```python
from build123d import *

# Parameters (mm, degrees)
ZAAWANSOWANYOTW_R1_START       = 2
ZAAWANSOWANYOTW_R1_DEPTH       = 3
ZAAWANSOWANYOTW_R1_2_OUTLINE_R = 1.1
ZAAWANSOWANYOTW_R1_2_DEPTH     = 2
SZKIC6_W                       = 8
SZKIC6_H                       = 3.2
SZKIC6_W_2                     = 7.6
SZKIC6_H_2                     = 2.8
DODANIE_WYCI_GNI_CIE1_DEPTH    = 2.6
WYTNIJ_WYCI_GNI_CIE1_REACH     = 30.598
SZKIC7_W                       = 7.2
SZKIC7_H                       = 1.5
DODANIE_WYCI_GNI_CIE2_DEPTH    = 2.4
ZAOKR_GLENIE1_R                = 0.1


# Read off the part's stored shape, not the designer's step: ZaawansowanyOtwór1
with BuildPart() as part:
    # Szkic1 → Obrót1 (revolve)
    with BuildSketch(Plane(origin=(0, 0, 0), x_dir=(0, 0, -1), z_dir=(1, 0, 0))):
        Polygon((0, 19), (-11.4, 19), (-11.5, 18.9), (-11.5, 0), (-6.2, 0), (-6.2, 2), (-9.5, 2), (-9.5, 13), (0, 13), align=None)
    revolve(axis=Axis((0, 22.266164505, 0), (0, -1, 0)))

    # ZaawansowanyOtwór1 outline → ZaawansowanyOtwór1 (cut)
    with BuildSketch(Plane(origin=(0, 0, 0), x_dir=(1, 0, 0), z_dir=(0, 1, 0)).offset(ZAAWANSOWANYOTW_R1_START)):
        with BuildLine():
            ThreePointArc((6.592725397, 6.840027181), (5.45, 9.439676901), (2.627274603, 9.129481265))
            ThreePointArc((2.627274603, 9.129481265), (4.75, 8.227241336), (6.592725397, 6.840027181))
        make_face()
        with BuildLine():
            ThreePointArc((-6.592725397, -6.840027181), (-5.45, -9.439676901), (-2.627274603, -9.129481265))
            ThreePointArc((-2.627274603, -9.129481265), (-4.75, -8.227241336), (-6.592725397, -6.840027181))
        make_face()
    extrude(amount=ZAAWANSOWANYOTW_R1_DEPTH, mode=Mode.SUBTRACT)

    # ZaawansowanyOtw_r1 2 outline → ZaawansowanyOtw_r1 2 (cut)
    with BuildSketch(Plane(origin=(0, 0, 0), x_dir=(1, 0, 0), z_dir=(0, 1, 0))):
        with Locations((4.25, 7.361215932)):
            Circle(ZAAWANSOWANYOTW_R1_2_OUTLINE_R)
        with Locations((-4.25, -7.361215932)):
            Circle(ZAAWANSOWANYOTW_R1_2_OUTLINE_R)
    extrude(amount=ZAAWANSOWANYOTW_R1_2_DEPTH, mode=Mode.SUBTRACT)

    # Szkic6 → Dodanie-wyciągnięcie1 (add)
    with BuildSketch(Plane(origin=(0, 19, 0), x_dir=(1, 0, 0), z_dir=(0, 1, 0))):
        with Locations((0, 4.9)):
            Rectangle(SZKIC6_W, SZKIC6_H)
        with Locations((0, 4.9)):
            Rectangle(SZKIC6_W_2, SZKIC6_H_2, mode=Mode.SUBTRACT)
    extrude(amount=DODANIE_WYCI_GNI_CIE1_DEPTH)

    # Szkic7 → Wytnij-wyciągnięcie1 (cut, up to next)
    with BuildSketch(Plane.XY.offset(-3.3), mode=Mode.PRIVATE) as wytnij_wyci_gni_cie1_sk1:
        with Locations((0, 20.85)):
            Rectangle(SZKIC7_W, SZKIC7_H)
    wytnij_wyci_gni_cie1_tool1 = extrude(wytnij_wyci_gni_cie1_sk1.sketch, amount=-WYTNIJ_WYCI_GNI_CIE1_REACH, mode=Mode.PRIVATE) & part.part
    add(wytnij_wyci_gni_cie1_tool1.solids().sort_by_distance((0, 20.85, -3.3))[0], mode=Mode.SUBTRACT)

    # Szkic8 → Dodanie-wyciągnięcie2 (add)
    with BuildSketch(Plane(origin=(0, 19, 0), x_dir=(1, 0, 0), z_dir=(0, 1, 0))):
        with BuildLine():
            Line((-2.95, 5.6), (-2.95, 5.4))
            ThreePointArc((-2.95, 5.4), (-3.1, 5.25), (-3.25, 5.4))
            Line((-3.25, 5.4), (-3.25, 5.6))
            ThreePointArc((-3.25, 5.6), (-3.1, 5.75), (-2.95, 5.6))
        make_face()
        with BuildLine():
            Line((-1.4, 5.6), (-1.4, 5.4))
            ThreePointArc((-1.4, 5.4), (-1.55, 5.25), (-1.7, 5.4))
            Line((-1.7, 5.4), (-1.7, 5.6))
            ThreePointArc((-1.7, 5.6), (-1.55, 5.75), (-1.4, 5.6))
        make_face()
        with BuildLine():
            Line((0.15, 5.6), (0.15, 5.4))
            ThreePointArc((0.15, 5.4), (0, 5.25), (-0.15, 5.4))
            Line((-0.15, 5.4), (-0.15, 5.6))
            ThreePointArc((-0.15, 5.6), (0, 5.75), (0.15, 5.6))
        make_face()
        with BuildLine():
            Line((1.7, 5.6), (1.7, 5.4))
            ThreePointArc((1.7, 5.4), (1.55, 5.25), (1.4, 5.4))
            Line((1.4, 5.4), (1.4, 5.6))
            ThreePointArc((1.4, 5.6), (1.55, 5.75), (1.7, 5.6))
        make_face()
        with BuildLine():
            Line((3.25, 5.6), (3.25, 5.4))
            ThreePointArc((3.25, 5.4), (3.1, 5.25), (2.95, 5.4))
            Line((2.95, 5.4), (2.95, 5.6))
            ThreePointArc((2.95, 5.6), (3.1, 5.75), (3.25, 5.6))
        make_face()
    extrude(amount=DODANIE_WYCI_GNI_CIE2_DEPTH)

    # Zaokrąglenie1
    zaokr_glenie1_edges = [part.edges().sort_by_distance(p)[0] for p in [
        (-1.55, 21.4, -5.75),
        (-1.7, 21.4, -5.5),
        (-1.55, 21.4, -5.25),
        (-1.4, 21.4, -5.5),
        (0, 21.4, -5.75),
        (-0.15, 21.4, -5.5),
        (0, 21.4, -5.25),
        (0.15, 21.4, -5.5),
        (1.55, 21.4, -5.75),
        (1.4, 21.4, -5.5),
        (1.55, 21.4, -5.25),
        (1.7, 21.4, -5.5),
        (3.1, 21.4, -5.75),
        (2.95, 21.4, -5.5),
        (3.1, 21.4, -5.25),
        (3.25, 21.4, -5.5),
        (-3.1, 21.4, -5.75),
        (-3.25, 21.4, -5.5),
        (-3.1, 21.4, -5.25),
        (-2.95, 21.4, -5.5),
    ]]
    fillet(zaokr_glenie1_edges, radius=ZAOKR_GLENIE1_R)


solid = part.part
```
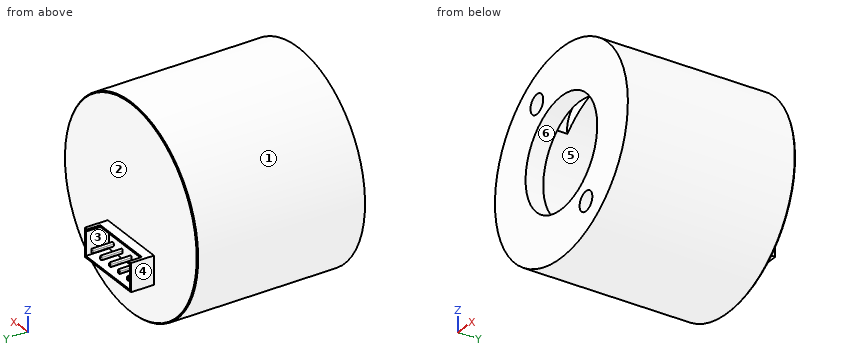
Here's how the part is built. I have some questions about the finished solid (model axes, mm). Face numbers are marked on the shaded views. A direction names the side the tool comes from. Coordinates: 2 decimals unless noted, no trailing zeros. Loops run counter-clockwise (first coordinate to the right, second up) from the corner with the lowest first, then second, coordinate; pieces in that order, holes last. Notation, with made-up numbers: (77.25, 21.25) -> (86.25, 21.25) arc R21 cw to (86.25, 26.25) -> close; hole circle Ø1 at (11, -34.5). An arc over 180 degrees is marked (long way). Return JSON: item names as keys, results as strings.
1) If we section it at B-B, the plane y = 3: Write out the boundary of the cut face in (x, z), then the cut area to 3 significant figures.
Results below:
{"outline": "circle Ø23 at (0, 0); hole (-6.59, 6.84) arc R9.5 ccw to (2.63, -9.13) arc R2.4 ccw to (6.59, -6.84) arc R9.5 ccw to (-2.63, 9.13) arc R2.4 ccw to start", "area": "122 mm²"}
2) If we section it at A-A, the plane z = 0: Write out the boundary of the cut face in (x, y), then the cut area to 3 significant figures.
Results below:
{"outline": "(-11.5, 0) -> (-6.2, 0) -> (-6.2, 2) -> (-9.5, 2) -> (-9.5, 13) -> (9.5, 13) -> (9.5, 2) -> (6.2, 2) -> (6.2, 0) -> (11.5, 0) -> (11.5, 18.9) -> (11.4, 19) -> (-11.4, 19) -> (-11.5, 18.9) -> close", "area": "203 mm²"}
3) If we section it at C-C, the plane y = 14.25: Write out the boundary of the cut face in (x, z).
Results below:
{"outline": "circle Ø23 at (0, 0)"}
4) Thinking about a two-plate mould opening in Z: for the marked faces 1, 2 and 3, which applies, +Z half, -Z half, draft (parallel to the pull), parting line (faces both ways), or undercut?
Results below:
{"face 1": "parting line", "face 2": "draft", "face 3": "undercut"}
5) I need wall thicknesses on line 1 (X direction, y = 10, z = 0); line 2 (Y direction, x = -7, z = -3.25); line 3 (Z direction, x = -4.25, y = 0.5). Which ranges of each line are inside material? Lowest first, please. Write a range as from..to.
Results below:
{"line 1": "-11.5..-9.5, 9.5..11.5", "line 2": "0..2, 13..19", "line 3": "-10.69..-4.51, 4.51..6.26, 8.46..10.69"}
6) For the marked faces 4, 5 and 6, which set-ups out of +Z, -Z, +X, -X, +Y, -Y let a thin tool reach every point of the face, with its end or its side?
Results below:
{"face 4": "+Z, -Z, -X, +Y", "face 5": "none", "face 6": "-Y"}
7) Will these pins go through, and if not, where does the flat tip stop? pin 1 (5 mm diameter, centred on x = 4.5, y = 18.5, fed in from +Z); pin 2 (1 mm diameter, centred on x = 4.5, z = -7.5, fed in from -Y); pin 3 (0.8 mm diameter, centred on y = 20, z = -5.5, fed in from -X).
Results below:
{"pin 1": "z = 11.32", "pin 2": "y = 13", "pin 3": "x = -4"}
8) If we section it at D-D, the plane y = 11: Write out the boundary of the cut face in (x, z), then the cut area to 3 significant figures.
Results below:
{"outline": "circle Ø23 at (0, 0); hole circle Ø19 at (0, 0)", "area": "132 mm²"}
